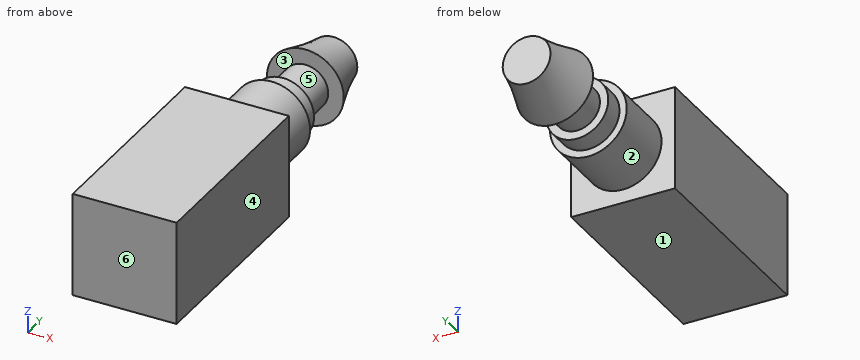
```python
from build123d import *

# Parameters (mm, degrees)
SKETCH1_R           = 1.85
BOSS_EXTRUDE1_DEPTH = 3.1
SKETCH2_R           = 1.5
BOSS_EXTRUDE2_DEPTH = 1
SKETCH3_R           = 1.1
BOSS_EXTRUDE3_DEPTH = 2
SKETCH6_W           = 5
SKETCH6_H           = 5
BOSS_EXTRUDE4_DEPTH = 10


with BuildPart() as part:
    # Sketch1 → Boss-Extrude1 (new body)
    with BuildSketch(Plane(origin=(0, 0, 0), x_dir=(1, 0, 0), z_dir=(0, 1, 0))):
        with Locations(Location((0, 0, 0), (0, 0, 90))):
            Circle(SKETCH1_R)
    extrude(amount=BOSS_EXTRUDE1_DEPTH)

    # Sketch2 → Boss-Extrude2 (add)
    with BuildSketch(Plane(origin=(0, 3.1, 0), x_dir=(1, 0, 0), z_dir=(0, 1, 0))):
        with Locations(Location((0, 0, 0), (0, 0, 270))):
            Circle(SKETCH2_R)
    extrude(amount=BOSS_EXTRUDE2_DEPTH)

    # Sketch3 → Boss-Extrude3 (add)
    with BuildSketch(Plane(origin=(0, 4.1, 0), x_dir=(1, 0, 0), z_dir=(0, 1, 0))):
        with Locations(Location((0, 0, 0), (0, 0, 270))):
            Circle(SKETCH3_R)
    extrude(amount=BOSS_EXTRUDE3_DEPTH)

    # Loft1: read off the stored shape, not the designer's step
    # Loft1: loft between two sections, ruled curve by curve
    loft1_from = [
        Edge.make_bspline([(0, 6.1, 1.85), (3.7, 6.1, 1.85), (3.7, 6.1, -1.85), (0, 6.1, -1.85), (-3.7, 6.1, -1.85), (-3.7, 6.1, 1.85), (0, 6.1, 1.85)], [0, 0, 0, 0, 0.5, 0.5, 0.5, 1, 1, 1, 1], 3, [1, 0.333333333, 0.333333333, 1, 0.333333333, 0.333333333, 1]),
    ]
    loft1_to = [
        Edge.make_bspline([(0.620465421, 8.6, 0.968257539), (2.556980499, 8.6, -0.272673303), (1.316049657, 8.6, -2.209188381), (-0.620465421, 8.6, -0.968257539), (-2.556980499, 8.6, 0.272673303), (-1.316049657, 8.6, 2.209188381), (0.620465421, 8.6, 0.968257539)], [0, 0, 0, 0, 0.5, 0.5, 0.5, 1, 1, 1, 1], 3, [1, 0.333333333, 0.333333333, 1, 0.333333333, 0.333333333, 1]),
    ]
    loft1 = Solid(Shell([*[Face.make_surface_from_curves(loft1_from[k], loft1_to[k]) for k in range(1)], Face(Wire(loft1_from)), Face(Wire(loft1_to))]))
    add(loft1)

    # Sketch6 → Boss-Extrude4 (add)
    with BuildSketch(Plane.XZ):
        Rectangle(SKETCH6_W, SKETCH6_H)
    extrude(amount=BOSS_EXTRUDE4_DEPTH)


solid = part.part
```
Source: CAD feature listing. Evaluate the final solid. Frame: model axes, mm. Face numbers are marked on the shaded views. A direction names the side the tool comes from. Coordinates: 2 decimals unless noted, no trailing zeros. Loops run counter-clockwise (first coordinate to the right, second up) from the corner with the lowest first, then second, coordinate; pieces in that order, holes last. Notation, with made-up numbers: M 49,-30.75 L 84,-30.75 A33 cw 84,3.25 Z; hole C 68.5,20 d9. An arc over 180 degrees is marked long. Use a Markdown table: item, result. Add a question column.
Q1. Section query A-A, the plane y = 2.5. Return loops of the section in (x, z), and give its area (3 significant figures).
Q2. Draft query along Y for the marked faces 4, 5 and 6. Return one class per face: pulls with the +Y half, pulls with the -Y half, needs draft (parallel to the pull), parting line crosses it, or undercut.
Q3. Access query for the marked faces 1, 2 and 3. Directions: +Z, -Z, +X, -X, +Y, -Y. A direction counts if a zero-diameter tool reaches every point of the face in a straight line with its end or side. Return the directions, or none.
Q4. Section query C-C, the plane z = 2.05. Return loops of the section in (x, y).
Q5. First-contact query: pin 1 (2 mm diameter, centred on x = -1, y = 3, fed in from -Z). Flat tip, straight axial feed; report the tip coordinate or a pass-through.
Q6. Section query B-B, the plane x = 2.25. Return loops of the section in (y, z), and give its area (3 significant figures).
Q7. Material intervals for L1, parallel to Y at x = -1.55, z = -1.95; L2, parallel to X at y = 1.25, z = -1.45, sorted ascending.
Result:
| question | item | result |
|---|---|---|
| 1 | outline | C 0,0 d3.7 |
| 1 | area | 10.8 mm2 |
| 2 | face 4 | needs draft |
| 2 | face 5 | undercut |
| 2 | face 6 | pulls with the -Y half |
| 3 | face 1 | -Z, +X, -X, +Y, -Y |
| 3 | face 2 | +Y |
| 3 | face 3 | none |
| 4 | outline | M -2.5,-10 L 2.5,-10 L 2.5,0 L -2.5,0 Z |
| 5 | pin 1 | stops at z = -1.85 |
| 6 | outline | M -10,-2.5 L 0,-2.5 L 0,2.5 L -10,2.5 Z |
| 6 | area | 50.0 mm2 |
| 7 | L1 | y = -10 to 0 |
| 7 | L2 | x = -1.15 to 1.15 |
